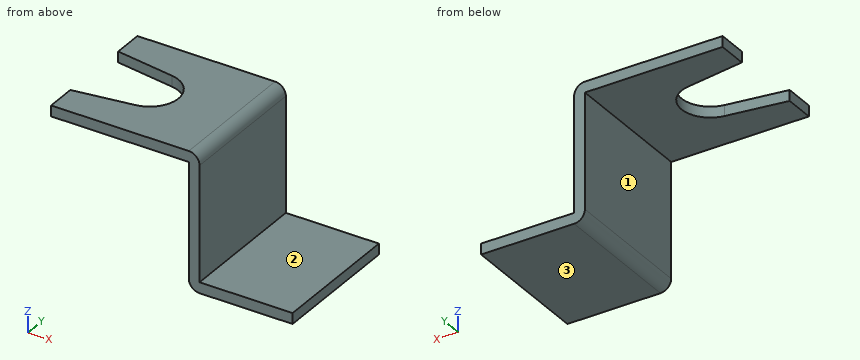
from build123d import *

# Parameters (mm, degrees)
F1_DEPTH = 25
F2_R     = 5.3407247833
F3_DEPTH = 25.3101193046
F5_DEPTH = 106
F6_DEPTH = 25.3101193046


# Not quite as in the source:
# - an extrude ends at something that could not be found from the text; its depth is read off the source's solid


with BuildPart() as f1:
    # F0 (on Front) → F1 (new body)
    with BuildSketch(Plane.XZ):
        with BuildLine():
            Line((-2, 0), (-58.1267029047, 0))
            Line((-58.1267029047, 0), (-58.1267029047, -2))
            Line((-58.1267029047, -2), (-2, -2))
            Line((-2, -2), (-2, -23.3091193046))
            ThreePointArc((-2, -23.3091193046), (-1.4142135624, -24.723332867), (0, -25.3091193046))
            Line((0, -25.3091193046), (17.2828252222, -25.3091193046))
            Line((17.2828252222, -25.3091193046), (17.2828252222, -23.3091193046))
            Line((17.2828252222, -23.3091193046), (0, -23.3091193046))
            Line((0, -23.3091193046), (0, -2))
            ThreePointArc((0, -2), (-0.5857864376, -0.5857864376), (-2, 0))
        make_face()
    extrude(amount=F1_DEPTH)

    # F2 (on face) → F3 (cut, through all)
    with BuildSketch(Plane.XY):
        with Locations((-17.279623447, -12.5)):
            Circle(F2_R)
    extrude(amount=-F3_DEPTH, mode=Mode.SUBTRACT)

    # F4 (on face) → F5 (cut, through all)
    with BuildSketch(Plane.XY):
        with BuildLine():
            Line((-27.5714416057, -5.5710808575), (-27.5714416057, 0))
            Line((-27.5714416057, 0), (-58.1267029047, 0))
            Line((-58.1267029047, 0), (-58.1267029047, -25))
            Line((-58.1267029047, -25), (-27.5714416057, -25))
            Line((-27.5714416057, -25), (-27.5714416057, -19.4289191425))
            Line((-27.5714416057, -19.4289191425), (-16.4945252417, -17.7827040443))
            ThreePointArc((-16.4945252417, -17.7827040443), (-22.6203482303, -12.5), (-16.4945252417, -7.2172959557))
            Line((-16.4945252417, -7.2172959557), (-27.5714416057, -5.5710808575))
        make_face()
    extrude(amount=F5_DEPTH, mode=Mode.SUBTRACT)

    # F4 (on face) → F6 (cut, through all)
    with BuildSketch(Plane.XY):
        with BuildLine():
            Line((-27.5714416057, -5.5710808575), (-27.5714416057, 0))
            Line((-27.5714416057, 0), (-58.1267029047, 0))
            Line((-58.1267029047, 0), (-58.1267029047, -25))
            Line((-58.1267029047, -25), (-27.5714416057, -25))
            Line((-27.5714416057, -25), (-27.5714416057, -19.4289191425))
            Line((-27.5714416057, -19.4289191425), (-16.4945252417, -17.7827040443))
            ThreePointArc((-16.4945252417, -17.7827040443), (-22.6203482303, -12.5), (-16.4945252417, -7.2172959557))
            Line((-16.4945252417, -7.2172959557), (-27.5714416057, -5.5710808575))
        make_face()
    extrude(amount=-F6_DEPTH, mode=Mode.SUBTRACT)


solid = f1.part
Verification items for the finished model (mm, model axes). Face numbers are marked on the shaded views. A direction names the side the tool comes from. Coordinates: 2 decimals unless noted, no trailing zeros. Order: outer loops, then holes, each group sorted by start corner. A loop starts at its lowest first (then second) coordinate and runs counter-clockwise, first axis right, second up. Notation, with made-up numbers: M -5,20.25 L 29,20.25 A27 cw 29,49.25 Z; hole C -17,54 d3. An arc over 180 degrees is marked long. One line per item, written item: value. Start each with the question number.
Item 1: Access from +Z, -Z, +X, -X, +Y, -Y to the whole of each face (thin tool, end or side, straight path). Record for the marked faces 1, 2 and 3.
Item 2: Sectioned sample at A-A on y = -20.5. Record the cut outline in (x, z), then the cut area to 3 significant figures.
Item 3: Thickness scan on probe 1 along X at (y, z) = (-22, -12.75); probe 2 along Z at (x, y) = (10.5, -5.75). Record the ranges inside material, lowest first.
Item 4: Depth check by flat-ended pin: P1, Ø2, axis at y = -3, z = -19.5, coming from the +X side; P2, Ø4, axis at y = -3, z = -13, coming from the -X side; P3, Ø12.5, axis at x = -11.5, y = -11, coming from the -Z side. Enter the tip coordinate at first touch or a pass-through.
Item 5: Sectioned sample at C-C on z = -7.5. Record the cut outline in (x, y).
Item 6: Sectioned sample at B-B on x = -20.5. Record the cut outline in (y, z), then the cut area to 3 significant figures.
Item 7: Sectioned sample at D-D on y = -11.25. Record the cut outline in (x, z).
Calculated:
1. face 1: -Z, -X, +Y, -Y
1. face 2: +Z, +X, +Y, -Y
1. face 3: -Z, +X, -X, +Y, -Y
2. outline: M -27.57,-2 L -2,-2 L -2,-23.31 A2 ccw 0,-25.31 L 17.28,-25.31 L 17.28,-23.31 L 0,-23.31 L 0,-2 A2 ccw -2,0 L -27.57,0 Z
2. area: 135 mm^2
3. probe 1: -2 to 0
3. probe 2: -25.31 to -23.31
4. P1: x = 0
4. P2: x = -2
4. P3: z = -2
5. outline: M -2,-25 L 0,-25 L 0,0 L -2,0 Z
6. outline: M -25,-2 L -18.38,-2 L -18.38,0 L -25,0 Z; M -6.62,-2 L 0,-2 L 0,0 L -6.62,0 Z
6. area: 26.5 mm^2
7. outline: M -12.09,-2 L -2,-2 L -2,-23.31 A2 ccw 0,-25.31 L 17.28,-25.31 L 17.28,-23.31 L 0,-23.31 L 0,-2 A2 ccw -2,0 L -12.09,0 Z
